The model under review builds one solid part; all positions refer to its coordinate system, in mm. Round coordinates to 2 decimals unless told otherwise and drop trailing zeros. Loops run counter-clockwise (first coordinate to the right, second up) from the corner with the lowest first, then second, coordinate; pieces in that order, holes last. Notation, with made-up numbers: M -16.75,22.5 L 39.25,22.5 A20 cw 39.25,42.5 Z; hole C 3,11 d9. An arc over 180 degrees is marked long. Answer as a JSON object with one key per item and string values. Group by question number.
Item 1: Consider section B-B (y = 604.5). Give the boundary of the cut face in (x, z), and give its area (3 significant figures).
Item 2: Consider section C-C (x = 0). State how many separate pieces and enclosed holes the cut face has, and give its area (3 significant figures).
Item 3: To check wall thickness, follow line 1 (Y direction, x = 0, z = -13.9); line 2 (Z direction, x = -12.5, y = 523). State the ranges of each line that lie inside material, in increasing order.
Item 4: Consider section A-A (z = -1). Give the boundary of the cut face in (x, y).
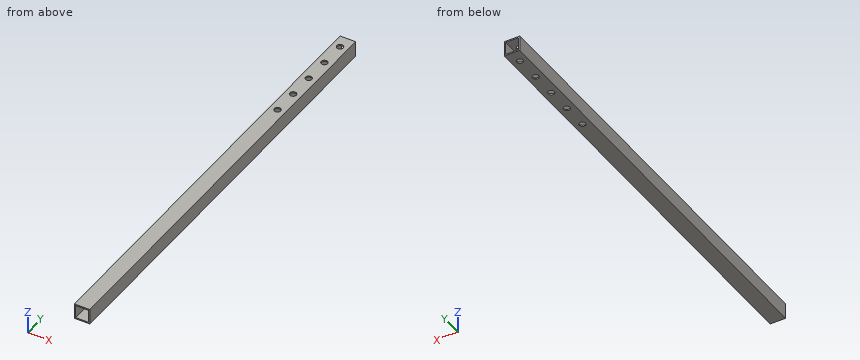
```python
from build123d import *

# Parameters (mm, degrees)
SKETCH1_W           = 30.48
SKETCH1_H           = 30.48
SKETCH1_W_2         = 25.4
SKETCH1_H_2         = 25.4
EXTRUDE_THIN1_DEPTH = 863.6
SKETCH2_R           = 6.35
CUT_EXTRUDE1_DEPTH  = 865.272091416
LPATTERN1_COUNT     = 5
LPATTERN1_PITCH     = 50.8


with BuildPart() as part:
    # Sketch1 → Extrude-Thin1 (new body)
    with BuildSketch(Plane(origin=(0, 0, 0), x_dir=(1, 0, 0), z_dir=(0, 1, 0))):
        Rectangle(SKETCH1_W, SKETCH1_H)
        Rectangle(SKETCH1_W_2, SKETCH1_H_2, mode=Mode.SUBTRACT)
    extrude(amount=EXTRUDE_THIN1_DEPTH)

    # Sketch2 → Cut-Extrude1 (cut, through all)
    with BuildSketch(Plane.XY.offset(15.24)):
        with Locations((0, 838.2)):
            Circle(SKETCH2_R)
    cut_extrude1 = extrude(amount=-CUT_EXTRUDE1_DEPTH, mode=Mode.SUBTRACT)

    # LPattern1: Cut-Extrude1 ×5
    with Locations(*[(0, -i * LPATTERN1_PITCH, 0) for i in range(1, LPATTERN1_COUNT)]):
        add(cut_extrude1, mode=Mode.SUBTRACT)


solid = part.part
```
Geometry results:
{
 "1": {"outline": "M -15.24,-15.24 L 15.24,-15.24 L 15.24,15.24 L -15.24,15.24 Z; hole M -12.7,-12.7 L 12.7,-12.7 L 12.7,12.7 L -12.7,12.7 Z", "area": "284 mm^2"},
 "2": {"separate pieces": "12", "enclosed holes": "0", "area": "4,060 mm^2"},
 "3": {"line 1": "y = 0 to 628.65, 641.35 to 679.45, 692.15 to 730.25, 742.95 to 781.05, 793.75 to 831.85, 844.55 to 863.6", "line 2": "z = -15.24 to -12.7, 12.7 to 15.24"},
 "4": {"outline": "M -15.24,0 L -12.7,0 L -12.7,863.6 L -15.24,863.6 Z; M 12.7,0 L 15.24,0 L 15.24,863.6 L 12.7,863.6 Z"}
}
